from build123d import *

# Parameters (mm, degrees)
FILLET_R = 2


with BuildPart() as part:
    # Sketch → Revolution (revolve)
    with BuildSketch(Plane.XZ):
        Polygon((0, 5), (13, 5), (13, 0), (10.5, 0), (11.2, -2), (10.5, -4), (11.2, -6), (10.5, -8), (11.2, -10), (10.5, -12), (9, -12), (9, 0), (0, 0), align=None)
    revolve(axis=Axis((0, 0, 0), (0, 0, 1)))

    # Fillet
    fillet_edges = [part.edges().sort_by_distance(p)[0] for p in [
        (-13, 0, 5),
    ]]
    fillet(fillet_edges, radius=FILLET_R)


solid = part.part
Verification items for the finished model (mm, model axes). A direction names the side the tool comes from. Coordinates: 2 decimals unless noted, no trailing zeros. Loops run counter-clockwise (first coordinate to the right, second up) from the corner with the lowest first, then second, coordinate; pieces in that order, holes last. Notation, with made-up numbers: (70, 59) -> (126, 59) arc R9 cw to (126, 71) -> close; hole circle Ø6 at (78, 73). An arc over 180 degrees is marked (long way). Write each question's results on one line, items separated by ' | '.
Item 1: Gauge pin test, flat ends, axial feed: pin 1 (6 mm diameter, centred on y = 7.5, z = -0.5, fed in from -X); pin 2 (5 mm diameter, centred on x = 8, z = -0.5, fed in from +Y); pin 3 (4 mm diameter, centred on x = 2.5, z = -9, fed in from +Y). Record the tip position at first contact, or that the pin passes through.
Found:
pin 1: stops at x = -12.18 | pin 2: stops at y = 11.76 | pin 3: stops at y = 11.17
Item 2: Mould release check, pull along X, two halves, no side actions. Record for faces 1 (the face through (-10.316, -7.91, 1.479)), 2 (the face through (0, 0, 5)), 3 (the face through (0, 0, 0)): +X half, -X half, draft (parallel to the pull), parting line (faces both ways), or undercut.
Found:
face 1: parting line | face 2: draft | face 3: undercut
Item 3: Section check A-A, the plane x = 0. Enter the section's corners in (y, z), plus the area to 3 significant figures.
Found:
outline: (-13, 0) -> (-10.5, 0) -> (-11.2, -2) -> (-10.5, -4) -> (-11.2, -6) -> (-10.5, -8) -> (-11.2, -10) -> (-10.5, -12) -> (-9, -12) -> (-9, 0) -> (9, 0) -> (9, -12) -> (10.5, -12) -> (11.2, -10) -> (10.5, -8) -> (11.2, -6) -> (10.5, -4) -> (11.2, -2) -> (10.5, 0) -> (13, 0) -> (13, 3) arc R2 ccw to (11, 5) -> (-11, 5) arc R2 ccw to (-13, 3) -> close | area: 173 mm2
Item 4: Material ranges on L1, parallel to Y at x = 0, z = -4; L2, parallel to Z at x = -1.25, y = -3.5; L3, parallel to Y at x = -0.25, z = 2, recorded low to high.
Found:
L1: y = -10.5 to -9, 9 to 10.5 | L2: z = 0 to 5 | L3: y = -13 to 13
Item 5: Section check D-D, the plane z = -7.5. Enter the section's corners in (x, y) (3 decimals).
Found:
outline: circle Ø21.35 at (0, 0); hole circle Ø18 at (0, 0)
Item 6: Section check C-C, the plane z = 1.75. Enter the section's corners in (x, y).
Found:
outline: circle Ø26 at (0, 0)
Item 7: Tool access check on faces 4 (the face through (-9, 6, 0)), 5 (the face through (-1.172, 8.923, -5.916)), 6 (the face through (8, 5, -12)). Record the directions out of +Z, -Z, +X, -X, +Y, -Y that give a thin tool (end or side, any length) a straight path to the whole face; none if there is none.
Found:
face 4: none | face 5: -Z | face 6: -Z, +X, -X, +Y, -Y
